from build123d import *

# Parameters (mm, degrees)
BOSS_EXTRUDE1_DEPTH     = 38.1
SKETCH2_R               = 3.175
CUT_EXTRUDE1_DEPTH      = 38.1
CUT_EXTRUDE3_REACH      = 79.512
SKETCH3_R               = 3.175
CUT_EXTRUDE4_DEPTH      = 75.882225236
CUT_EXTRUDE4_DEPTH_BACK = 75.882225236
CHAMFER1_SIZE           = 2.54


with BuildPart() as part:
    # Sketch1 → Boss-Extrude1 (new body)
    with BuildSketch(Plane(origin=(0, 0, 0), x_dir=(1, 0, 0), z_dir=(0, 1, 0))):
        Polygon((0, 0), (0, 46.0375), (39.6875, 46.0375), (39.6875, 50.8), (-4.7625, 50.8), (-4.7625, 0), align=None)
    extrude(amount=BOSS_EXTRUDE1_DEPTH)

    # Sketch2 → Cut-Extrude1 (cut)
    with BuildSketch(Plane(origin=(0, 0, -50.8), x_dir=(-1, 0, 0), z_dir=(0, 0, -1))):
        with Locations((-26.338386991, 20.92691832)):
            Circle(SKETCH2_R)
        with Locations((-7.9375, 15.996415511)):
            Circle(SKETCH2_R)
    extrude(amount=-CUT_EXTRUDE1_DEPTH, mode=Mode.SUBTRACT)

    # Sketch3 → Cut-Extrude3 (cut, up to next)
    with BuildSketch(Plane.ZY.offset(4.7625), mode=Mode.PRIVATE) as cut_extrude3_sk1:
        with Locations((-12.7, 19.05)):
            Circle(SKETCH3_R)
    cut_extrude3_tool1 = extrude(cut_extrude3_sk1.sketch, amount=-CUT_EXTRUDE3_REACH, mode=Mode.PRIVATE) & part.part
    # Sketch3 → Cut-Extrude3 (cut, up to next)
    with BuildSketch(Plane.ZY.offset(4.7625), mode=Mode.PRIVATE) as cut_extrude3_sk2:
        with Locations((-31.75, 19.05)):
            Circle(SKETCH3_R)
    cut_extrude3_tool2 = extrude(cut_extrude3_sk2.sketch, amount=-CUT_EXTRUDE3_REACH, mode=Mode.PRIVATE) & part.part
    add(cut_extrude3_tool1.solids().sort_by_distance((-4.7625, 19.05, -12.7))[0], mode=Mode.SUBTRACT)
    add(cut_extrude3_tool2.solids().sort_by_distance((-4.7625, 19.05, -31.75))[0], mode=Mode.SUBTRACT)

    # Sketch4 → Cut-Extrude4 (cut, two sides: drawn at the far end of the back side and taken through both)
    with BuildSketch(Plane(origin=(0, 0, -50.8), x_dir=(-1, 0, 0), z_dir=(0, 0, -1)).offset(-CUT_EXTRUDE4_DEPTH_BACK)):
        Polygon((3.41421458, 160.857788706), (-29.478635768, 38.1), (-39.6875, 0), (-72.580350349, -122.757788706), (-318.095927761, -56.972088009), (-242.101362833, 226.643489404), align=None)
    extrude(amount=CUT_EXTRUDE4_DEPTH + CUT_EXTRUDE4_DEPTH_BACK, mode=Mode.SUBTRACT)

    # Chamfer1
    chamfer1_edges = [part.edges().sort_by_distance(p)[0] for p in [
        (0, 19.05, -15.875),
        (0, 19.05, -34.925),
    ]]
    chamfer(chamfer1_edges, length=CHAMFER1_SIZE)


solid = part.part
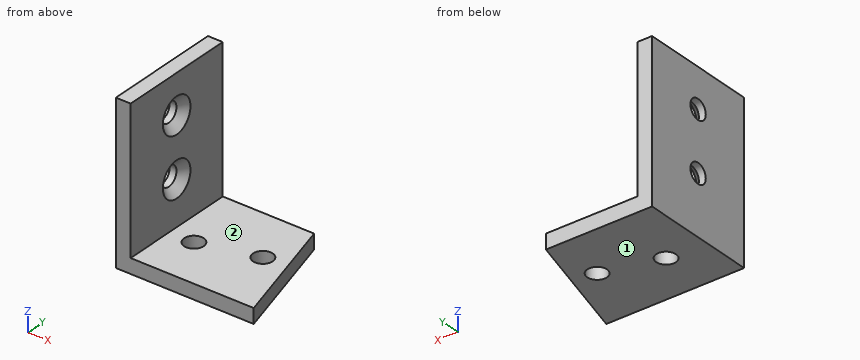
Check sheet for the modelled part. Datum: model origin and axes. Units: mm. Face numbers are marked on the shaded views. A direction names the side the tool comes from. Round coordinates to 2 decimals unless told otherwise and drop trailing zeros. Loops run counter-clockwise (first coordinate to the right, second up) from the corner with the lowest first, then second, coordinate; pieces in that order, holes last. Notation, with made-up numbers: (17.5, 73) -> (43.5, 73) arc R29 ccw to (43.5, 100) -> close; hole circle Ø5 at (21, 88). An arc over 180 degrees is marked (long way). Put each result on its own line as item: value. Start each with the question number.
1. Section check D-D (y = 26). Enter the section's corners in (x, z).
2. Scan lines: probe 1 along Y at (x, z) = (-4.15, -12.7) (3 decimals); probe 2 along X at (y, z) = (19.5, -39); probe 3 along Z at (x, y) = (28.5, 15). Record each from-to range of solid material in increasing order.
3. Gauge pin test, flat ends, axial feed: pin 1 (19 mm diameter, centred on x = 16, y = 15.5, fed in from +Z); pin 2 (1 mm diameter, centred on y = 7.5, z = -29, fed in from +X); pin 3 (10 mm diameter, centred on y = 19.05, z = -31.75, fed in from +X) (3 decimals). Record the tip position at first contact, or that the pin passes through.
4. Section check A-A (z = -12.7). Enter the section's corners in (x, y) (1 decimal), plus the area to 3 significant figures.
5. Access from +Z, -Z, +X, -X, +Y, -Y to the whole of each face (thin tool, end or side, straight path). Record for the marked faces 1 and 2.
6. Section check C-C (x = 14.5). Enter the section's corners in (y, z).
7. Section check B-B (x = 25). Enter the section's corners in (y, z).
Findings:
1. outline: (-4.76, -50.8) -> (32.72, -50.8) -> (32.72, -46.04) -> (0, -46.04) -> (0, 0) -> (-4.76, 0) -> close
2. probe 1: y = 0 to 15.875, 22.225 to 38.1
2. probe 2: x = -4.76 to 0
2. probe 3: z = -50.8 to -46.04
3. pin 1: stops at z = -46.04
3. pin 2: stops at x = 0
3. pin 3: stops at x = -0.715
4. outline: (-4.8, 0) -> (0, 0) -> (0, 13.3) -> (-2.5, 15.9) -> (-4.8, 15.9) -> close; (-4.8, 22.2) -> (-2.5, 22.2) -> (0, 24.8) -> (0, 38.1) -> (-4.8, 38.1) -> close
4. area: 145 mm^2
5. face 1: -Z, +X, -X, +Y, -Y
5. face 2: +Z, +X, +Y, -Y
6. outline: (0, -50.8) -> (38.1, -50.8) -> (38.1, -46.04) -> (0, -46.04) -> close
7. outline: (0, -50.8) -> (18.05, -50.8) -> (18.05, -46.04) -> (0, -46.04) -> close; (23.81, -50.8) -> (38.1, -50.8) -> (38.1, -46.04) -> (23.81, -46.04) -> close
